Geometry check sheet. Reference: the model listing, model coordinates, mm. A direction names the side the tool comes from. Give positions to 0.01 mm unless a question says otherwise; leave off trailing zeros. Order: outer loops, then holes, each group sorted by start corner. A loop starts at its lowest first (then second) coordinate and runs counter-clockwise, first axis right, second up.
from build123d import *

# Parameters (mm, degrees)
BOSS_EXTRUDE3_DEPTH = 3


with BuildPart() as part:
    # Sketch3 → Boss-Extrude3 (new body)
    with BuildSketch(Plane.XY):
        with BuildLine():
            Line((1.5, -40.798266812), (1.5, -17.877938214))
            Line((1.5, -17.877938214), (-1.5, -17.877938214))
            Line((-1.5, -17.877938214), (-1.5, -40.798266812))
            Line((-1.5, -40.798266812), (-5.5, -40.798266812))
            Line((-5.5, -40.798266812), (-5.5, -17.877938214))
            Line((-5.5, -17.877938214), (-8.5, -17.877938214))
            Line((-8.5, -17.877938214), (-8.5, -40.798266812))
            Line((-8.5, -40.798266812), (-13.869579038, -40.798266812))
            ThreePointArc((-13.869579038, -40.798266812), (-12.587739972, -19.904581661), (-13.963477054, 0.983130949))
            Line((-13.963477054, 0.983130949), (-11.963477054, 0.983130949))
            Line((-11.963477054, 0.983130949), (-11.963477054, 3.983130949))
            Line((-11.963477054, 3.983130949), (-14.381577939, 3.983130949))
            ThreePointArc((-14.381577939, 3.983130949), (-14.622945439, 5.553795951), (-14.879439279, 7.122061786))
            ThreePointArc((-14.879439279, 7.122061786), (-14.579260447, 7.711309245), (-13.976966099, 7.984368613))
            Line((-13.976966099, 7.984368613), (-2.75, 8.982321155))
            ThreePointArc((-2.75, 8.982321155), (-2.498879462, 9.076941447), (-2.33284853, 9.287768993))
            ThreePointArc((-2.33284853, 9.287768993), (-1.875511855, 11.141722585), (-2, 13.047189315))
            add(Edge.make_bspline(
                [(-1.5, 27.249432049), (-17.245966692, 21.162756592), (-2, 13.047189315)],
                knots=[3.417819284, 3.417819284, 3.417819284, 5.911016773, 5.911016773, 5.911016773], degree=2, weights=[1, 0.318548271, 1]))
            Line((-1.5, 27.249432049), (-1.5, 19.749432049))
            Line((-1.5, 19.749432049), (1.5, 19.749432049))
            Line((1.5, 19.749432049), (1.5, 27.249432049))
            add(Edge.make_bspline(
                [(2, 13.047189315), (17.245966692, 21.162756592), (1.5, 27.249432049)],
                knots=[0.372168534, 0.372168534, 0.372168534, 2.865366023, 2.865366023, 2.865366023], degree=2, weights=[1, 0.318548271, 1]))
            ThreePointArc((2, 13.047189315), (1.875511855, 11.141722585), (2.33284853, 9.287768993))
            ThreePointArc((2.33284853, 9.287768993), (2.498879462, 9.076941447), (2.75, 8.982321155))
            Line((2.75, 8.982321155), (13.976966099, 7.984368613))
            ThreePointArc((13.976966099, 7.984368613), (14.579260447, 7.711309245), (14.879439279, 7.122061786))
            ThreePointArc((14.879439279, 7.122061786), (14.622945439, 5.553795951), (14.381577939, 3.983130949))
            Line((14.381577939, 3.983130949), (11.963477054, 3.983130949))
            Line((11.963477054, 3.983130949), (11.963477054, 0.983130949))
            Line((11.963477054, 0.983130949), (13.963477054, 0.983130949))
            ThreePointArc((13.963477054, 0.983130949), (12.587739972, -19.904581661), (13.869579038, -40.798266812))
            Line((13.869579038, -40.798266812), (8.5, -40.798266812))
            Line((8.5, -40.798266812), (8.5, -17.877938214))
            Line((8.5, -17.877938214), (5.5, -17.877938214))
            Line((5.5, -17.877938214), (5.5, -40.798266812))
            Line((5.5, -40.798266812), (1.5, -40.798266812))
        make_face()
    extrude(amount=BOSS_EXTRUDE3_DEPTH)


solid = part.part
Item 1: Scan lines: L1, parallel to X at y = -32, z = 2.55; L2, parallel to X at y = -30, z = 2.65; L3, parallel to Y at x = 12.25, z = 2. Record each from-to range of solid material in increasing order.
Reported:
L1: x = -13 to -8.5, -5.5 to -1.5, 1.5 to 5.5, 8.5 to 13
L2: x = -12.87 to -8.5, -5.5 to -1.5, 1.5 to 5.5, 8.5 to 12.87
L3: y = -40.8 to 0.98, 3.98 to 8.14
Item 2: Gauge pin test, flat ends, axial feed: pin 1 (1.5 mm diameter, centred on y = -27.5, z = 1.5, fed in from +X); pin 2 (1.5 mm diameter, centred on x = 0.5, z = 2, fed in from -Y); pin 3 (1.5 mm diameter, centred on y = 2, z = 1.5, fed in from +X). Record the tip position at first contact, or that the pin passes through.
Reported:
pin 1: stops at x = 12.78
pin 2: stops at y = -17.88
pin 3: stops at x = 11.96
Item 3: Sectioned sample at C-C (y = 11). Enter the section's corners in (x, z).
Reported:
outline: (-1.89, 0) - (1.89, 0) - (1.89, 3) - (-1.89, 3) - close
Item 4: Draft check along X on faces 1 (the flat face through (-8.5, -29, 1)), 2 (the flat face through (0, -17.878, 1)), 3 (the cylindrical face through (-14.62, 5.53, 1.48)), 4 (the flat face through (0, -6, 3)). Enter one of: released by +X, released by -X, zero draft, split by the parting line, or undercut.
Reported:
face 1: undercut
face 2: undercut
face 3: released by -X
face 4: zero draft
Item 5: Set-up check for faces 5 (the flat face through (0, -6, 0)), 6 (the flat face through (11.963, 3, 1)), 7 (the flat face through (1.5, 23, 1)), 8 (the flat face through (-13, 0.983, 1)), 9 (the flat face through (-5.5, -29, 1)): record each of +Z, -Z, +X, -X, +Y, -Y from which the full face is reachable in a straight line by a thin tool's end or side.
Reported:
face 5: -Z, +X, -X, +Y, -Y
face 6: +Z, -Z, +X
face 7: +Z, -Z, +Y
face 8: +Z, -Z, -X
face 9: +Z, -Z, -Y
Item 6: Sectioned sample at A-A (x = 13.25). Enter the section's corners in (y, z).
Reported:
outline: (-40.8, 0) - (-35.04, 0) - (-35.04, 3) - (-40.8, 3) - close; (-5.51, 0) - (0.98, 0) - (0.98, 3) - (-5.51, 3) - close; (3.98, 0) - (8.05, 0) - (8.05, 3) - (3.98, 3) - close
Item 7: Sectioned sample at B-B (y = -30.5). Enter the section's corners in (x, z).
Reported:
outline: (-12.9, 0) - (-8.5, 0) - (-8.5, 3) - (-12.9, 3) - close; (-5.5, 0) - (-1.5, 0) - (-1.5, 3) - (-5.5, 3) - close; (1.5, 0) - (5.5, 0) - (5.5, 3) - (1.5, 3) - close; (8.5, 0) - (12.9, 0) - (12.9, 3) - (8.5, 3) - close
Item 8: Sectioned sample at D-D (x = 7.5). Enter the section's corners in (y, z), and give its area (3 significant figures).
Reported:
outline: (-17.88, 0) - (8.56, 0) - (8.56, 3) - (-17.88, 3) - close
area: 79.3 mm2
